```python
from build123d import *

# Parameters (mm, degrees)
SKETCH1_W           = 50.8
SKETCH1_H           = 25.4
SKETCH1_W_2         = 44.45
SKETCH1_H_2         = 19.05
BOSS_EXTRUDE1_DEPTH = 98.552
SKETCH2_R           = 6.35
CUT_EXTRUDE1_DEPTH  = 114.746633814


with BuildPart() as part:
    # Sketch1 → Boss-Extrude1 (new body)
    with BuildSketch(Plane.XY):
        with Locations((25.4, 12.7)):
            Rectangle(SKETCH1_W, SKETCH1_H)
        with Locations((25.4, 12.7)):
            Rectangle(SKETCH1_W_2, SKETCH1_H_2, mode=Mode.SUBTRACT)
    extrude(amount=BOSS_EXTRUDE1_DEPTH)

    # Sketch2 → Cut-Extrude1 (cut, through all)
    with BuildSketch(Plane.XZ):
        with Locations(Location((25.4, 12.7, 0), (0, 0, 270))):
            Circle(SKETCH2_R)
    extrude(amount=-CUT_EXTRUDE1_DEPTH, mode=Mode.SUBTRACT)


solid = part.part
```
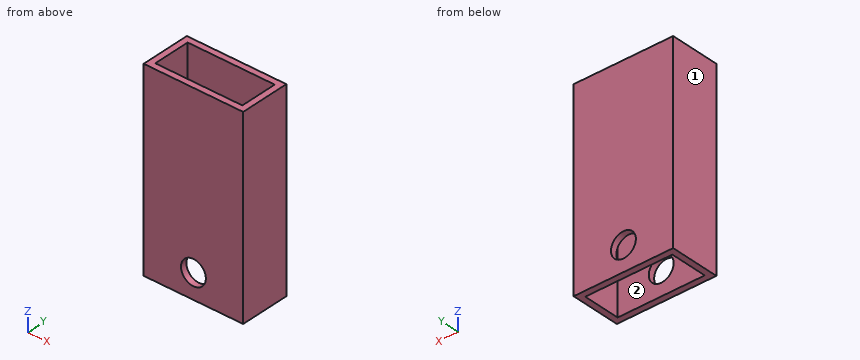
Part model, mm, in its own coordinate system. Face numbers are marked on the shaded views. A direction names the side the tool comes from. Give positions to 0.01 mm unless a question says otherwise; leave off trailing zeros. Write each loop counter-clockwise with the first axis right and the second up, starting at its lowest first coordinate (ties: lowest second). Pieces come first, ordered by that corner, then holes. Notation, with made-up numbers: (18.25, -14.75) -> (22.25, -14.75) arc R18 cw to (22.25, 4.25) -> close; hole circle Ø5 at (-18.75, -18.5). An arc over 180 degrees is marked (long way). Put each result on its own line as item: value. Start each with the question number.
Item 1: Pin check, flat tip, straight feed: pin 1 Ø11.5 at (x, z) = (25.4, 12.7) entering from +Y. Stop position of the tip, or through.
Item 2: Which spindle directions (+Z, -Z, +X, -X, +Y, -Y) get a long thin tool onto all of the face, cutting with end or side? Do the marked faces 1 and 2. Say none if no direction does.
Item 3: Wall check: L1, parallel to X at y = 23.1, z = 12.7; L2, parallel to Y at x = 20, z = 37 (3 decimals); L3, parallel to X at y = 11.25, z = 65 (3 decimals). Give the ranges that are in metal, low to high. Write a range as [from, to].
Item 4: Cut at A-A (y = 7.25). List the corners of the cut face in (x, z) (3 decimals), then the cut area to 3 significant figures.
Item 5: Cut at D-D (z = 12.7). List the corners of the cut face in (x, y) (3 decimals).
Item 6: Cut at B-B (z = 64). List the corners of the cut face in (x, y) (3 decimals), then the cut area to 3 significant figures.
Item 7: Cut at C-C (x = 40). List the corners of the cut face in (y, z) (3 decimals), then the cut area to 3 significant figures.
Answer list:
1. pin 1: passes through
2. face 1: +Z, -Z, -X, +Y, -Y
2. face 2: +Z, -Z
3. L1: x = [0, 19.05], [31.75, 50.8]
3. L2: y = [0, 3.175], [22.225, 25.4]
3. L3: x = [0, 3.175], [47.625, 50.8]
4. outline: (0, 0) -> (3.175, 0) -> (3.175, 98.552) -> (0, 98.552) -> close; (47.625, 0) -> (50.8, 0) -> (50.8, 98.552) -> (47.625, 98.552) -> close
4. area: 626 mm2
5. outline: (0, 0) -> (19.05, 0) -> (19.05, 3.175) -> (3.175, 3.175) -> (3.175, 22.225) -> (19.05, 22.225) -> (19.05, 25.4) -> (0, 25.4) -> close; (31.75, 0) -> (50.8, 0) -> (50.8, 25.4) -> (31.75, 25.4) -> (31.75, 22.225) -> (47.625, 22.225) -> (47.625, 3.175) -> (31.75, 3.175) -> close
6. outline: (0, 0) -> (50.8, 0) -> (50.8, 25.4) -> (0, 25.4) -> close; hole (3.175, 3.175) -> (47.625, 3.175) -> (47.625, 22.225) -> (3.175, 22.225) -> close
6. area: 444 mm2
7. outline: (0, 0) -> (3.175, 0) -> (3.175, 98.552) -> (0, 98.552) -> close; (22.225, 0) -> (25.4, 0) -> (25.4, 98.552) -> (22.225, 98.552) -> close
7. area: 626 mm2
